Input: part model. Units: mm. Frame: model coordinates. Face numbers are marked on the shaded views. A direction names the side the tool comes from. Coordinates: 2 decimals unless noted, no trailing zeros. Write each loop counter-clockwise with the first axis right and the second up, starting at its lowest first coordinate (ties: lowest second). Pieces come first, ordered by that corner, then holes. Notation, with made-up numbers: (-10.5, 20) - (45.5, 20) arc R14 ccw to (45.5, 43) - close; hole circle Ø8 at (77.5, -28.5). An arc over 180 degrees is marked (long way). One line per question, with ' | ' between items. Start each with the question number.
1) Section query B-B on z = 25. Return loops of the section in (x, y).
2) Line query: line 1 (X direction, y = 1, z = -25); line 2 (Y direction, x = 0.5, z = -26.5); line 3 (Y direction, x = 7.75, z = 12). Output: solid intervals per line, ascending.
3) Draft query along Y for the marked faces 6, 7 and 8. Return one class per face: released by +Y, released by -Y, zero draft, split by the parting line, or undercut.
4) Section query A-A on z = -25. Return loops of the section in (x, y).
5) Reachability of the marked faces 1, 2, 3, 4 and 5 from +Z, -Z, +X, -X, +Y, -Y: full face, straight path, thin tool, end or side. Return the list, or none.
6) First-contact query: P1, Ø5.5, axis at x = -5.05, z = -25, coming from the -Y side; P2, Ø6, axis at x = 4, y = -8.5, coming from the +Z side; P3, Ø4.5, axis at x = -0.5, z = -26, coming from the +Y side; P4, Ø2.5, axis at x = -5.05, z = 25, coming from the -Y side. Flat tips, straight axial feed; report the tip coordinate or a pass-through.
7) Section query D-D on z = 4. Return loops of the section in (x, y).
8) Section query C-C on y = 7. Return loops of the section in (x, z).
```python
from build123d import *

# Parameters (mm, degrees)
SKETCH_1_W          = 19.4
SKETCH_1_H          = 7.7
SKETCH_1_R          = 2.05
SKETCH_1_H_2        = 40
EXTRUDE_1_DEPTH     = 2.5
SKETCH_1_3_W        = 19.4
SKETCH_1_3_H        = 40
EXTRUDE_2_DEPTH     = 28.4
EXTRUDE_START       = 2.5
SKETCH_1_4_W        = 19.4
SKETCH_1_4_H        = 40
EXTRUDE_3_DEPTH     = 7.5
SKETCH_2_R          = 2.925
EXTRUDE_4_DEPTH     = 6.1
SKETCH_4_2_R        = 4
EXTRUDE_5_DEPTH     = 1
SKETCH_6_R          = 7
SKETCH_7_R          = 5.25
SKETCH_8_R          = 1.5
CUT_EXTRUDE_1_DEPTH = 6.1
CUT_EXTRUDE_START   = -4
SKETCH_9_R          = 1.5
CUT_EXTRUDE_2_DEPTH = 4
SKETCH_10_W         = 8
SKETCH_10_H         = 6
EXTRUDE_6_DEPTH     = 2
SKETCH_11_W         = 5.5
SKETCH_11_H         = 4
EXTRUDE_7_DEPTH     = 10


with BuildPart() as part:
    # 스케치1 → 보스-돌출1 (new body)
    # profile 1 of 3: a face of its own
    with BuildSketch(Plane(origin=(0, 0, 0), x_dir=(1, 0, 0), z_dir=(0, 1, 0))):
        with Locations((0, 23.85)):
            Rectangle(SKETCH_1_W, SKETCH_1_H)
        with Locations(Location((-5.05, 25, 0), (0, 0, 270))):
            Circle(SKETCH_1_R, mode=Mode.SUBTRACT)
        with Locations(Location((5.05, 25, 0), (0, 0, 270))):
            Circle(SKETCH_1_R, mode=Mode.SUBTRACT)
    # profile 2 of 3: a face of its own
    with BuildSketch(Plane(origin=(0, 0, 0), x_dir=(1, 0, 0), z_dir=(0, 1, 0))):
        Rectangle(SKETCH_1_W, SKETCH_1_H_2)
    # profile 3 of 3: a face of its own
    with BuildSketch(Plane(origin=(0, 0, 0), x_dir=(1, 0, 0), z_dir=(0, 1, 0))):
        with Locations((0, -23.85)):
            Rectangle(SKETCH_1_W, SKETCH_1_H)
        with Locations(Location((-5.05, -25, 0), (0, 0, 270))):
            Circle(SKETCH_1_R, mode=Mode.SUBTRACT)
        with Locations(Location((5.05, -25, 0), (0, 0, 270))):
            Circle(SKETCH_1_R, mode=Mode.SUBTRACT)
    extrude(amount=EXTRUDE_1_DEPTH)

    # 스케치1<3> → 보스-돌출2 (add)
    with BuildSketch(Plane(origin=(0, 0, 0), x_dir=(1, 0, 0), z_dir=(0, 1, 0))):
        Rectangle(SKETCH_1_3_W, SKETCH_1_3_H)
    extrude(amount=-EXTRUDE_2_DEPTH)

    # 스케치1<4> → 보스-돌출3 (add)
    with BuildSketch(Plane(origin=(0, 0, 0), x_dir=(1, 0, 0), z_dir=(0, 1, 0)).offset(EXTRUDE_START)):
        Rectangle(SKETCH_1_4_W, SKETCH_1_4_H)
    extrude(amount=EXTRUDE_3_DEPTH)

    # 스케치2 → 보스-돌출4 (add)
    with BuildSketch(Plane(origin=(0, 10, 0), x_dir=(1, 0, 0), z_dir=(0, 1, 0))):
        with Locations(Location((0, 10.125, 0), (0, 0, 90))):
            Circle(SKETCH_2_R)
    extrude(amount=EXTRUDE_4_DEPTH)

    # 로프트1: read off the stored shape, not the designer's step
    # 로프트1: loft between two sections, ruled curve by curve
    loft_1_from = [
        Edge.make_bspline([(1.462551233, -28.4, -3.279494621), (-12.228459525, -28.4, -0.354392156), (-15.15356199, -28.4, -14.045402913), (-1.462551233, -28.4, -16.970505379), (12.228459525, -28.4, -19.895607844), (15.15356199, -28.4, -6.204597087), (1.462551233, -28.4, -3.279494621)], [0, 0, 0, 0, 0.5, 0.5, 0.5, 1, 1, 1, 1], 3, [1, 0.333333333, 0.333333333, 1, 0.333333333, 0.333333333, 1]),
    ]
    loft_1_to = [
        Edge.make_bspline([(2.267005586, -31.4, -6.829444557), (-4.3241053, -31.4, -2.295433386), (-8.858116471, -31.4, -8.886544271), (-2.267005586, -31.4, -13.420555443), (4.3241053, -31.4, -17.954566614), (8.858116471, -31.4, -11.363455729), (2.267005586, -31.4, -6.829444557)], [0, 0, 0, 0, 0.5, 0.5, 0.5, 1, 1, 1, 1], 3, [1, 0.333333333, 0.333333333, 1, 0.333333333, 0.333333333, 1]),
    ]
    loft_1 = Solid(Shell([*[Face.make_surface_from_curves(loft_1_from[k], loft_1_to[k]) for k in range(1)], Face(Wire(loft_1_from)), Face(Wire(loft_1_to))]))
    add(loft_1)

    # 스케치4<2> → 보스-돌출5 (add)
    with BuildSketch(Plane(origin=(0, -31.4, 0), x_dir=(-1, 0, 0), z_dir=(0, -1, 0))):
        with Locations(Location((0, 10.125, 0), (0, 0, 235.476))):
            Circle(SKETCH_4_2_R)
    extrude(amount=EXTRUDE_5_DEPTH)

    # 스케치6 → 로프트2 section 0
    with BuildSketch(Plane(origin=(0, 10, 0), x_dir=(1, 0, 0), z_dir=(0, 1, 0))):
        with Locations((0, 10.125)):
            Circle(SKETCH_6_R)
    # 스케치7 → 로프트2 section 1
    with BuildSketch(Plane(origin=(0, 12, 0), x_dir=(1, 0, 0), z_dir=(0, 1, 0))):
        with Locations((0, 10.125)):
            Circle(SKETCH_7_R)
    loft()

    # 스케치8 → 컷-돌출1 (cut)
    with BuildSketch(Plane(origin=(0, 16.1, 0), x_dir=(1, 0, 0), z_dir=(0, 1, 0))):
        with Locations(Location((0, 10.125, 0), (0, 0, 270))):
            Circle(SKETCH_8_R)
    extrude(amount=-CUT_EXTRUDE_1_DEPTH, mode=Mode.SUBTRACT)

    # 스케치9 → 컷-돌출2 (cut)
    with BuildSketch(Plane.XZ.offset(32.4).offset(CUT_EXTRUDE_START)):
        with Locations(Location((0, -10.125, 0), (0, 0, 90))):
            Circle(SKETCH_9_R)
    extrude(amount=CUT_EXTRUDE_2_DEPTH, mode=Mode.SUBTRACT)

    # 스케치10 → 보스-돌출6 (add)
    with BuildSketch(Plane(origin=(0, 0, -20), x_dir=(-1, 0, 0), z_dir=(0, 0, -1))):
        with Locations((0, -20.4)):
            Rectangle(SKETCH_10_W, SKETCH_10_H)
    extrude(amount=EXTRUDE_6_DEPTH)

    # 스케치11 → 보스-돌출7 (add)
    with BuildSketch(Plane(origin=(0, 0, -22), x_dir=(-1, 0, 0), z_dir=(0, 0, -1))):
        with Locations((0, -20.4)):
            Rectangle(SKETCH_11_W, SKETCH_11_H)
    extrude(amount=EXTRUDE_7_DEPTH)


solid = part.part
```
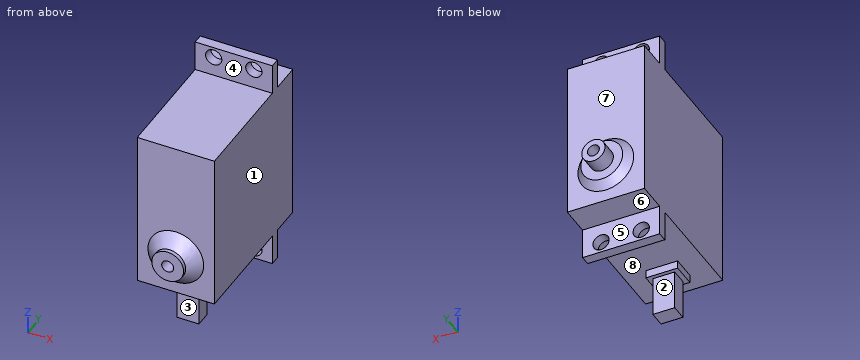
Answer key:
1) outline: (-9.7, 0) - (-7.1, 0) - (-7.1, 2.5) - (-9.7, 2.5) - close; (-3, 0) - (3, 0) - (3, 2.5) - (-3, 2.5) - close; (7.1, 0) - (9.7, 0) - (9.7, 2.5) - (7.1, 2.5) - close
2) line 1: -9.7 to -7.1, -3 to 3, 7.1 to 9.7 | line 2: -22.4 to -18.4, 0 to 2.5 | line 3: -28.4 to 10
3) face 6: zero draft | face 7: released by +Y | face 8: undercut
4) outline: (-9.7, 0) - (-7.1, 0) - (-7.1, 2.5) - (-9.7, 2.5) - close; (-3, 0) - (3, 0) - (3, 2.5) - (-3, 2.5) - close; (-2.75, -22.4) - (2.75, -22.4) - (2.75, -18.4) - (-2.75, -18.4) - close; (7.1, 0) - (9.7, 0) - (9.7, 2.5) - (7.1, 2.5) - close
5) face 1: +Z, -Z, +X, +Y, -Y | face 2: -Z, +X, -X | face 3: -Z, +X, -X, -Y | face 4: +Z, +X, -X, -Y | face 5: -Z, +X, -X, +Y
6) P1: y = -22.4 | P2: z = 20 | P3: y = 2.5 | P4: through
7) outline: (-9.7, -28.4) - (9.7, -28.4) - (9.7, 10) - (-9.7, 10) - close
8) outline: (-9.7, -20) - (9.7, -20) - (9.7, 20) - (-9.7, 20) - close
